Autodesk Inventor part; units mm, degrees
ref_plane "Work Plane1" through (0, 0, 0) normal (0, 0, 1) x (1, 0, 0)
ref_plane "Work Plane2" through (-137.8458, 0, 0) normal (0, 1, 0) x (1, 0, 0)
ref_plane "YZ Plane" through (0, 0, 0) normal (1, 0, 0) x (0, 1, 0)
ref_plane "Work Plane1" through (0, 0, 0) normal (0, 0, 1) x (1, 0, 0)
sketch "Sketch1" plane through (0, 0, 0) normal (0, 0, 1) x (1, 0, 0)
  line L0 (-77.8391, 0) -> (-108.8361, 0)
  line L1 (-108.8361, -33.02) -> (-108.8361, 0)
  line L2 (-77.8391, -33.02) -> (-108.8361, -33.02)
  line L3 (-77.8391, -33.02) -> (-77.8391, 0)
  line L4 (-152.4, 0) -> (0, 0) construction
  line L5 (-152.4, 0) -> (-152.4, 6.35) construction
  line L6 (0, 0) -> (0, 6.35) construction
  line L7 (-152.4, 0) -> (0, 0)
  line L8 (0, 0) -> (0, -101.6)
  line L9 (0, -101.6) -> (-152.4, -101.6)
  line L10 (-152.4, -101.6) -> (-152.4, 0)
  line L11 (-137.8458, 6.35) -> (-137.8458, 0)
  line L12 (-141.5542, 6.35) -> (-141.5542, 0)
  line L13 (-14.5542, 6.35) -> (-14.5542, 0)
  line L14 (-10.8458, 6.35) -> (-10.8458, 0)
  line L15 (-141.5542, 0) -> (-137.8458, 0)
  line L16 (-137.8458, 0) -> (-137.8458, -12.7)
  line L17 (-137.8458, -12.7) -> (-141.5542, -12.7)
  line L18 (-141.5542, -12.7) -> (-141.5542, 0)
  line L19 (-14.5542, 0) -> (-10.8458, 0)
  line L20 (-10.8458, 0) -> (-10.8458, -12.7)
  line L21 (-10.8458, -12.7) -> (-14.5542, -12.7)
  line L22 (-14.5542, -12.7) -> (-14.5542, 0)
  line L23 (-16.637, -5.7726) -> (-8.763, -5.7726)
  line L24 (-8.763, -5.7726) -> (-8.763, -8.5666)
  line L25 (-8.763, -8.5666) -> (-16.637, -8.5666)
  line L26 (-16.637, -8.5666) -> (-16.637, -5.7726)
  line L27 (-143.637, -5.7726) -> (-135.763, -5.7726)
  line L28 (-135.763, -5.7726) -> (-135.763, -8.5666)
  line L29 (-135.763, -8.5666) -> (-143.637, -8.5666)
  line L30 (-143.637, -8.5666) -> (-143.637, -5.7726)
  line L31 (-152.4, -50.8) -> (0, -50.8) construction
  line L32 (-137.8458, -107.95) -> (-137.8458, -101.6)
  line L33 (-141.5542, -107.95) -> (-141.5542, -101.6)
  line L34 (-14.5542, -107.95) -> (-14.5542, -101.6)
  line L35 (-10.8458, -107.95) -> (-10.8458, -101.6)
  line L36 (-141.5542, -101.6) -> (-137.8458, -101.6)
  line L37 (-137.8458, -101.6) -> (-137.8458, -88.9)
  line L38 (-137.8458, -88.9) -> (-141.5542, -88.9)
  line L39 (-141.5542, -88.9) -> (-141.5542, -101.6)
  line L40 (-14.5542, -101.6) -> (-10.8458, -101.6)
  line L41 (-10.8458, -101.6) -> (-10.8458, -88.9)
  line L42 (-10.8458, -88.9) -> (-14.5542, -88.9)
  line L43 (-14.5542, -88.9) -> (-14.5542, -101.6)
  line L44 (-16.637, -95.8274) -> (-8.763, -95.8274)
  line L45 (-8.763, -95.8274) -> (-8.763, -93.0334)
  line L46 (-8.763, -93.0334) -> (-16.637, -93.0334)
  line L47 (-16.637, -93.0334) -> (-16.637, -95.8274)
  line L48 (-143.637, -95.8274) -> (-135.763, -95.8274)
  line L49 (-135.763, -95.8274) -> (-135.763, -93.0334)
  line L50 (-135.763, -93.0334) -> (-143.637, -93.0334)
  line L51 (-143.637, -93.0334) -> (-143.637, -95.8274)
  dimension "d0" = 101.6
  dimension "d1" = 12.7
  dimension "d2" = 7.874
  dimension "d3" = 2.794
  dimension "d6" = 2.0828
  dimension "d7" = 2.0828
  dimension "d8" = 7.874
  dimension "d9" = 2.0828
  dimension "d10" = 2.0828
ref_plane "Work Plane2" through (-137.8458, 0, 0) normal (0, 1, 0) x (1, 0, 0)
sketch "Sketch2" plane through (-137.8458, 0, 0) normal (0, 1, 0) x (1, 0, 0)
  line L0 (35.8892, 0) -> (10.4892, 0)
  line L1 (10.4892, 0) -> (10.4892, 6.35)
  line L2 (10.4892, 6.35) -> (35.8892, 6.35)
  line L3 (35.8892, 6.35) -> (35.8892, 0)
  line L4 (112.0892, 0) -> (86.6892, 0)
  line L5 (112.0892, 6.35) -> (112.0892, 0)
  line L6 (86.6892, 6.35) -> (112.0892, 6.35)
  line L7 (86.6892, 0) -> (86.6892, 6.35)
  point P0 (137.8458, 0)
extrude "Extrusion2" add sketch "Sketch2" along normal blind 6.35
extrude "Extrusion3" add sketch "Sketch1" against normal blind 6.35 contours L3 L2 L1 L0 | L7 L22 L23 L26 L25 L21 L20 L24 L8 L9 L41 L44 L45 L46 L42 L43 L47 L37 L48 L49 L50 L38 L39 L51 L10 L18 L27 L30 L29 L17 L16 L28 L1 L2 L3
sketch "Sketch3" plane through (-137.8458, -101.6, 0) normal (0, -1, 0) x (1, 0, 0)
  line L0 (35.8892, 0) -> (35.8892, -6.35)
  line L1 (35.8892, -6.35) -> (10.4892, -6.35)
  line L2 (10.4892, -6.35) -> (10.4892, 0)
  line L3 (10.4892, 0) -> (35.8892, 0)
  line L4 (112.0892, 0) -> (112.0892, -6.35)
  line L5 (112.0892, -6.35) -> (86.6892, -6.35)
  line L6 (86.6892, -6.35) -> (86.6892, 0)
  line L7 (86.6892, 0) -> (112.0892, 0)
  point P0 (137.8458, 0)
extrude "Extrusion4" add sketch "Sketch3" along normal blind 6.35
equation "\"d6\" = d7"
equation "\"d9\" = d10"
properties part number "baseBoxShortSideRB01"
Build history of the part. All positions in model axes, mm. A direction names the side the tool comes from. Give positions to 0.01 mm unless a question says otherwise; leave off trailing zeros. Order: outer loops, then holes, each group sorted by start corner. A loop starts at its lowest first (then second) coordinate and runs counter-clockwise, first axis right, second up. Notation, with made-up numbers: M 62,53 L 83,53 A22 ccw 83,86 Z; hole C -19.5,-8.5 d5. An arc over 180 degrees is marked long. Put each result on its own line as item: value.
Item 1: Probe line 1 (X direction, y = -2, z = -1.5); line 2 (X direction, y = -103, z = -4.5); line 3 (Y direction, x = -67, z = -3). List the from-to ranges inside material, lowest first. Write a range as [from, to].
From the geometry:
line 1: x = [-152.4, -141.55], [-137.85, -14.55], [-10.85, 0]
line 2: x = [-127.36, -101.96], [-51.16, -25.76]
line 3: y = [-101.6, 0]
Item 2: 3-axis set-ups, long thin cutter, end or side, ignore diameter. For faces 1 (the flat face through (-133, -101.6, -3)), 2 (the flat face through (-133, 0, -3)), 3 (the flat face through (-101.957, -105, -3)), 4 (the flat face through (-20, 0, -3)), 5 (the flat face through (-51.157, 3, -3)): which of +Z, -Z, +X, -X, +Y, -Y reach the whole face in a straight line?
From the geometry:
face 1: +Z, -Z, -X, -Y
face 2: +Z, -Z, -X, +Y
face 3: +Z, -Z, -Y
face 4: +Z, -Z, +X, +Y
face 5: +Z, -Z, +Y
Item 3: Slice it at A-A, the plane y = -100. Write the cut outline in (x, z).
From the geometry:
outline: M -152.4,-6.35 L -141.55,-6.35 L -141.55,0 L -152.4,0 Z; M -137.85,-6.35 L -14.55,-6.35 L -14.55,0 L -137.85,0 Z; M -10.85,-6.35 L 0,-6.35 L 0,0 L -10.85,0 Z
Item 4: Two-plate mould, pull along X, no slides. Class faces 6 (the flat face through (-76, 0, -3)), 7 (the flat face through (-115, 6.35, -3)), 8 (the flat face through (-25.757, -105, -3)): +X half, -X half, draft (parallel to the pull), parting line (faces both ways), or undercut.
From the geometry:
face 6: undercut
face 7: draft
face 8: +X half
Item 5: Slice it at B-B, the plane x = -61. Write the cut outline in (y, z), plus the area to 3 significant figures.
From the geometry:
outline: M -101.6,-6.35 L 0,-6.35 L 0,0 L -101.6,0 Z
area: 645 mm2
Item 6: Flat gauge pins, fed straight in: pin 1 Ø2.5 at (x, z) = (-136.5, -1.5) entering from -Y; pin 2 Ø3 at (x, z) = (-140.5, -2.5) entering from +Y; pin 3 Ø1.9 at (y, z) = (-105.5, -4.5) entering from -X. Where does each tip first touch, or does it go through?
From the geometry:
pin 1: stops at y = -101.6
pin 2: stops at y = 0
pin 3: stops at x = -127.36
